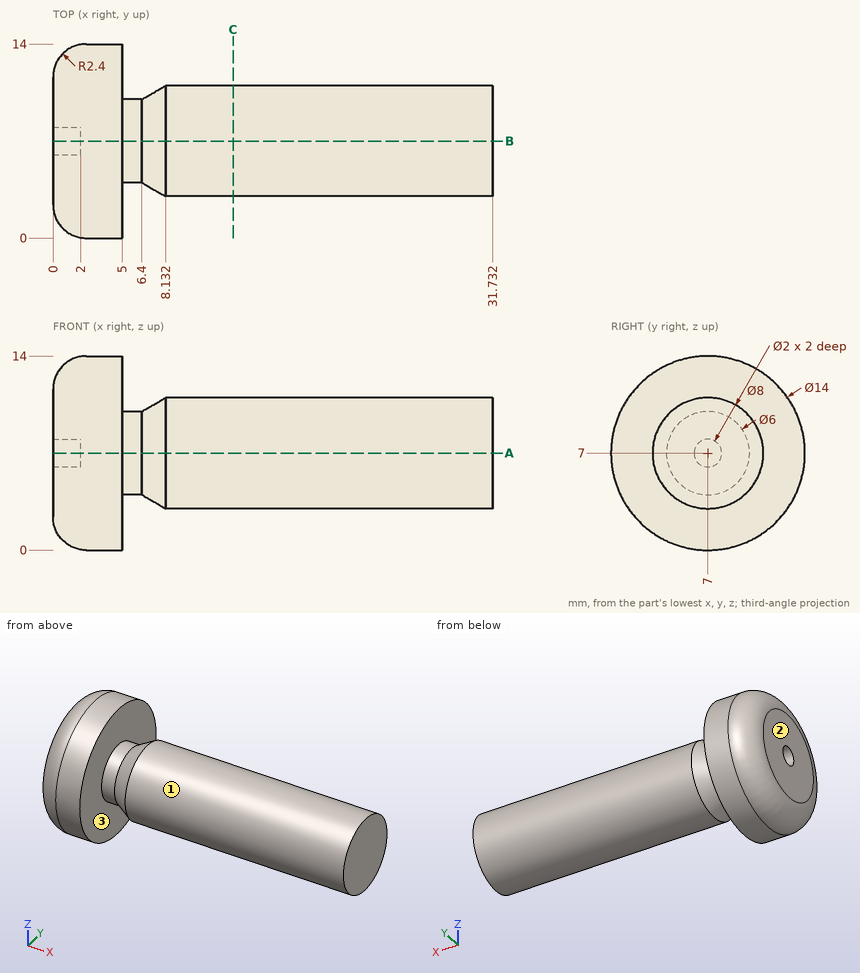
Geometry: see drawing. Coordinates: mm, zero at the bounding-box minimum. A direction names the side the tool comes from. Give positions to 0.01 mm unless a question says otherwise; leave off trailing zeros. Write each loop counter-clockwise with the first axis right and the second up, starting at its lowest first coordinate (ties: lowest second). Pieces come first, ordered by that corner, then holes. Notation, with made-up numbers: (30.5, 12.5) -> (44.5, 12.5) arc R33 cw to (44.5, 42.5) -> close; hole circle Ø2 at (89, -16). An arc over 180 degrees is marked (long way). Use one line per item in the form item = value. Start each with the question number.
1) Section query A-A on z = 7. Return the cut outline in (x, y).
2) Set-up query: the marked faces 1, 2 and 3. Return all of +Z, -Z, +X, -X, +Y, -Y with unobstructed straight access to the full face (end or side cutting, diameter ignored); none if empty.
3) Pin query (flat end, axial travel): pin 1 (2 mm diameter, centred on x = 21, y = 5.5, fed in from +Z); pin 2 (3 mm diameter, centred on x = 20.5, y = 10.5, fed in from -Z); pin 3 (8 mm diameter, centred on x = 15.5, z = 11.5, fed in from -Y). Return the tip coordinate at first contact, or that it passes through.
4) Section query C-C on x = 13. Return the cut outline in (y, z), then the cut area to 3 significant figures.
5) Ray query, probe 1 along X at (y, z) = (11, 6); probe 2 along Z at (x, y) = (1.5, 7) (1 decimal); probe 3 along X at (y, z) = (4.25, 5.5). Return the intervals inside material, ascending. Write a range as from..to.
Outcome:
q1.outline = (0, 2.4) arc R2.4 ccw to (2.4, 0) -> (5, 0) -> (5, 4) -> (6.4, 4) -> (8.13, 3) -> (31.73, 3) -> (31.73, 11) -> (8.13, 11) -> (6.4, 10) -> (5, 10) -> (5, 14) -> (2.4, 14) arc R2.4 ccw to (0, 11.6) -> (0, 8) -> (2, 8) -> (2, 6) -> (0, 6) -> close
q2.face_1 = +X
q2.face_2 = +Z, -Z, -X, +Y, -Y
q2.face_3 = none
q3.pin_1 = 10.97
q3.pin_2 = 3.54
q3.pin_3 = 3.03
q4.outline = circle Ø8 at (7, 7)
q4.area = 50.3 mm^2
q5.probe_1 = 0..5
q5.probe_2 = 0.2..6, 8..13.8
q5.probe_3 = 0..5, 6.63..31.73
